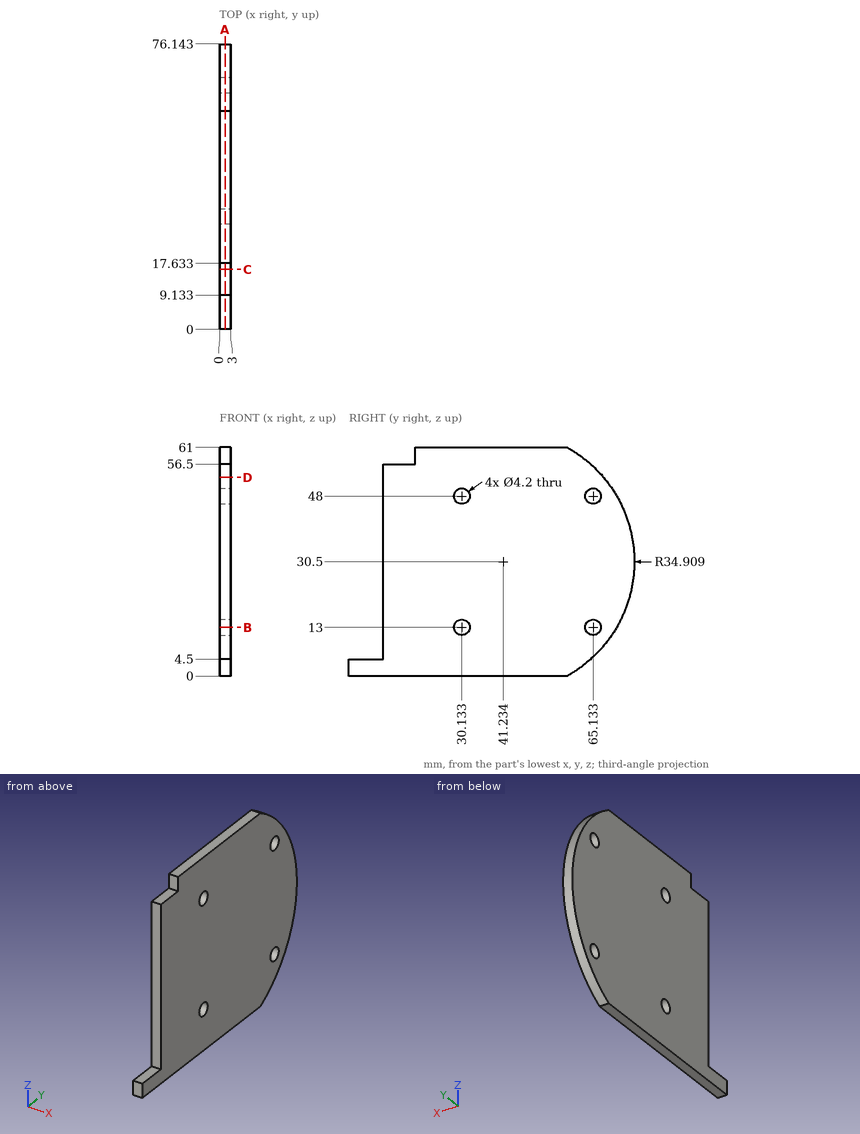
Part print with two shaded views. Sizes in mm from the minimum x, y, z corner. Round coordinates to 2 decimals unless told otherwise and drop trailing zeros. Write each loop counter-clockwise with the first axis right and the second up, starting at its lowest first coordinate (ties: lowest second). Pieces come first, ordered by that corner, then holes. Notation, with made-up numbers: M 58,-28 L 105,-28 A5 cw 105,-21 Z; hole C 41,73 d10. An arc over 180 degrees is marked long. Put each result on its own line as item: value. Start each with the question number.
1) Saw through at C-C, the plane y = 16. Write the cut outline in (x, z).
2) Drill centre lines: probe 1 along Z at (x, y) = (1.05, 31); probe 2 along Z at (x, y) = (2.25, 29); probe 3 along Y at (x, z) = (1.5, 48). Where is each one in solid material? Low to high. Write a range as [from, to].
3) Saw through at A-A, the plane x = 1.45. Write the cut outline in (y, z) (1 decimal), and give its area (3 significant figures).
4) Pin check, flat tips, straight feed: pin 1 Ø1.5 at (x, y) = (1.5, 14.5) entering from +Z; pin 2 Ø1.5 at (x, z) = (2.5, 47.5) entering from +Y; pin 3 Ø3.5 at (y, z) = (30.13, 48) entering from -X; pin 4 Ø1 at (x, z) = (1, 24.5) entering from +Y. Stop position of each tip, or through.
5) Saw through at D-D, the plane z = 53. Write the cut outline in (x, y) (1 decimal).
6) Saw through at B-B, the plane z = 13. Write the cut outline in (x, y), and give its area (3 significant figures).
Resolved:
1. outline: M 0,0 L 3,0 L 3,56.5 L 0,56.5 Z
2. probe 1: [0, 11.09], [14.91, 46.09], [49.91, 61]
2. probe 2: [0, 11.23], [14.77, 46.23], [49.77, 61]
2. probe 3: [9.13, 28.03], [32.23, 63.03], [67.23, 71.44]
3. outline: M 0,0 L 58.2,0 A34.9 ccw 58.2,61 L 17.6,61 L 17.6,56.5 L 9.1,56.5 L 9.1,4.5 L 0,4.5 Z; hole C 30.1,13 d4.2; hole C 30.1,48 d4.2; hole C 65.1,13 d4.2; hole C 65.1,48 d4.2
3. area: 3,720 mm²
4. pin 1: z = 56.5
4. pin 2: y = 72.13
4. pin 3: through
4. pin 4: y = 75.71
5. outline: M 0,9.1 L 3,9.1 L 3,67.9 L 0,67.9 Z
6. outline: M 0,9.13 L 3,9.13 L 3,28.03 L 0,28.03 Z; M 0,32.23 L 3,32.23 L 3,63.03 L 0,63.03 Z; M 0,67.23 L 3,67.23 L 3,71.44 L 0,71.44 Z
6. area: 162 mm²
